Answer from the drawing. Dimensions are ordinates in mm from the lowest x, y and z of the part. A direction names the side the tool comes from. Coordinates: 2 decimals unless noted, no trailing zeros. Loops run counter-clockwise (first coordinate to the right, second up) from the corner with the lowest first, then second, coordinate; pieces in that order, holes last.
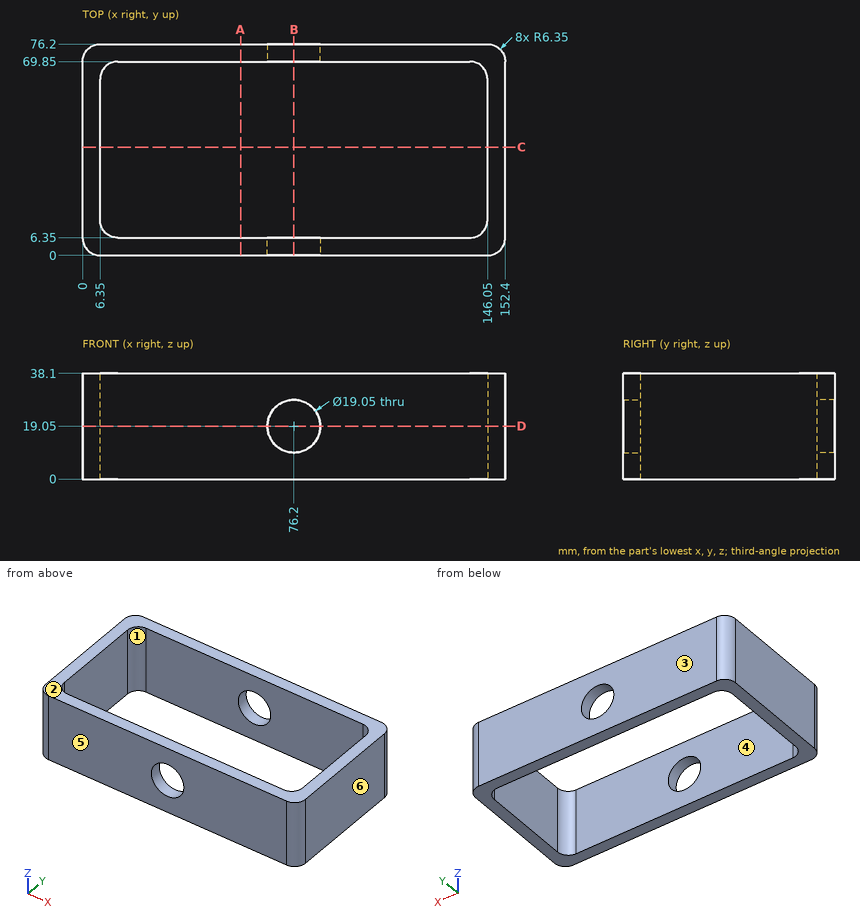
Item 1: A cutting plane is placed at C-C on y = 39. Determine the outline of the cut face in (x, z), then the cut area to 3 significant figures.
Numbers:
outline: (0, 0) - (6.35, 0) - (6.35, 38.1) - (0, 38.1) - close; (146.05, 0) - (152.4, 0) - (152.4, 38.1) - (146.05, 38.1) - close
area: 484 mm2
Item 2: Determine the mould class of the marked faces 3, 4, 5 and 6 for opening direction Y: released by +Y, released by -Y, zero draft, split by the parting line, or undercut.
Numbers:
face 3: released by +Y
face 4: undercut
face 5: released by -Y
face 6: zero draft
Item 3: A cutting plane is placed at D-D on z = 19.05. Determine the outline of the cut face in (x, y) (3 decimals).
Numbers:
outline: (0, 6.35) arc R6.35 ccw to (6.35, 0) - (66.675, 0) - (66.675, 6.35) - (12.7, 6.35) arc R6.35 cw to (6.35, 12.7) - (6.35, 63.5) arc R6.35 cw to (12.7, 69.85) - (66.675, 69.85) - (66.675, 76.2) - (6.35, 76.2) arc R6.35 ccw to (0, 69.85) - close; (85.725, 0) - (146.05, 0) arc R6.35 ccw to (152.4, 6.35) - (152.4, 69.85) arc R6.35 ccw to (146.05, 76.2) - (85.725, 76.2) - (85.725, 69.85) - (139.7, 69.85) arc R6.35 cw to (146.05, 63.5) - (146.05, 12.7) arc R6.35 cw to (139.7, 6.35) - (85.725, 6.35) - close
Item 4: A cutting plane is placed at A-A on x = 57. Determine the outline of the cut face in (y, z), then the cut area to 3 significant figures.
Numbers:
outline: (0, 0) - (6.35, 0) - (6.35, 38.1) - (0, 38.1) - close; (69.85, 0) - (76.2, 0) - (76.2, 38.1) - (69.85, 38.1) - close
area: 484 mm2
Item 5: Given pin 1 (10 mm diameter, centred on y = 41, z = 20, fed in from -X), flat-ended and moving along its own axis, determine where the tip first touches the part or whether it passes through.
Numbers:
pin 1: stops at x = 0
Item 6: Which of the six approach directions +Z, -Z, +X, -X, +Y, -Y give full straight-line access (tool end or side, diameter ignored) to the marked faces 1 and 2?
Numbers:
face 1: +Z, -Z
face 2: +Z, +X, -X, +Y, -Y
Item 7: Find the intervals of material crossed by line 1 along Z through (x, y) = (76, 3); line 2 along Y through (x, z) = (89, 16); line 3 along X through (y, z) = (62, 13.5), in increasing order.
Numbers:
line 1: z = 0 to 9.53, 28.57 to 38.1
line 2: y = 0 to 6.35, 69.85 to 76.2
line 3: x = 0 to 6.35, 146.05 to 152.4
Item 8: A cutting plane is placed at B-B on x = 76.2. Determine the outline of the cut face in (y, z) (3 decimals), then the cut area to 3 significant figures.
Numbers:
outline: (0, 0) - (6.35, 0) - (6.35, 9.525) - (0, 9.525) - close; (0, 28.575) - (6.35, 28.575) - (6.35, 38.1) - (0, 38.1) - close; (69.85, 0) - (76.2, 0) - (76.2, 9.525) - (69.85, 9.525) - close; (69.85, 28.575) - (76.2, 28.575) - (76.2, 38.1) - (69.85, 38.1) - close
area: 242 mm2
